from build123d import *

# Parameters (mm, degrees)
F0_W         = 166.2
F0_H         = 100.6
F1_DEPTH     = 5.96
F2_DEPTH     = 0.7
F3_W         = 15
F3_H         = 8
F4_DEPTH     = 2.5
F5_T4_DEPTH  = 33.7168298797
F5_T9_DEPTH  = 33.7168298797
F5_T14_DEPTH = 33.7168298797
F5_T19_DEPTH = 33.7168298797
F5_T24_DEPTH = 33.7168298797
F5_T29_DEPTH = 33.7168298797
F5_T34_DEPTH = 33.7168298797
F5_T39_DEPTH = 33.7168298797
F6_D         = 2.5
F6_DEPTH     = 2.501


# Not quite as in the source:
# - a fillet or chamfer that OpenCascade refuses, or shapes differently, is made with other operations: its cross-section is extruded or revolved along the edge and cut away or added


with BuildPart() as f1:
    # F0 (on Front) → F1 (new body)
    with BuildSketch(Plane.XZ):
        with Locations((-1.49, -1.55)):
            Rectangle(F0_W, F0_H)
    extrude(amount=F1_DEPTH)

    # F0 (on Front) → F2 (join)
    with BuildSketch(Plane.XZ):
        with BuildLine():
            ThreePointArc((-96.48, -47.5), (-94.1720014358, -53.0720014358), (-88.6, -55.38))
            Line((-88.6, -55.38), (88.6, -55.38))
            ThreePointArc((88.6, -55.38), (94.1720014357, -53.0720014357), (96.48, -47.5))
            Line((96.48, -47.5), (96.48, 47.5))
            ThreePointArc((96.48, 47.5), (94.1720014358, 53.0720014358), (88.6, 55.38))
            Line((88.6, 55.38), (-88.6, 55.38))
            ThreePointArc((-88.6, 55.38), (-94.1720014357, 53.0720014357), (-96.48, 47.5))
            Line((-96.48, 47.5), (-96.48, -47.5))
        make_face()
        with Locations((-1.49, -1.55)):
            Rectangle(F0_W, F0_H, mode=Mode.SUBTRACT)
    extrude(amount=F2_DEPTH)

    # F3 (on face) → F4 (join)
    with BuildSketch(Plane.XZ.offset(5.96)):
        with Locations((-64.59, 33.8)):
            Rectangle(F3_W, F3_H)
        with Locations((-64.59, -31.85)):
            Rectangle(F3_W, F3_H)
        with Locations((61.61, -31.85)):
            Rectangle(F3_W, F3_H)
        with Locations((61.61, 33.8)):
            Rectangle(F3_W, F3_H)
    extrude(amount=F4_DEPTH)

    # F5: chamfer of 5 on 8 edges, made by hand


with BuildPart() as f5_tool2:
    # F5_s3 → F5_t4 (new body)
    with BuildSketch(Plane.XY.offset(50.6584149398)):
        Polygon((-72.09, -3.46), (-67.09, -8.46), (-72.09, -8.46), align=None)
    extrude(amount=-F5_T4_DEPTH)

    split(bisect_by=Plane.XZ.offset(5.96), keep=Keep.TOP)


with BuildPart() as f1_1:
    add(f1.part)

    # F5_t1: cut F5_tool2
    add(f5_tool2.part, mode=Mode.SUBTRACT)


with BuildPart() as f5_tool7:
    # F5_s8 → F5_t9 (new body)
    with BuildSketch(Plane.XY.offset(16.9415850602)):
        Polygon((-57.09, -3.46), (-62.09, -8.46), (-57.09, -8.46), align=None)
    extrude(amount=F5_T9_DEPTH)

    split(bisect_by=Plane.XZ.offset(5.96), keep=Keep.TOP)


with BuildPart() as f1_2:
    add(f1_1.part)

    # F5_t6: cut F5_tool7
    add(f5_tool7.part, mode=Mode.SUBTRACT)


with BuildPart() as f5_tool12:
    # F5_s13 → F5_t14 (new body)
    with BuildSketch(Plane.XY.offset(-14.9915850602)):
        Polygon((-72.09, -3.46), (-67.09, -8.46), (-72.09, -8.46), align=None)
    extrude(amount=-F5_T14_DEPTH)

    split(bisect_by=Plane.XZ.offset(5.96), keep=Keep.TOP)


with BuildPart() as f1_3:
    add(f1_2.part)

    # F5_t11: cut F5_tool12
    add(f5_tool12.part, mode=Mode.SUBTRACT)


with BuildPart() as f5_tool17:
    # F5_s18 → F5_t19 (new body)
    with BuildSketch(Plane.XY.offset(-48.7084149398)):
        Polygon((-57.09, -3.46), (-62.09, -8.46), (-57.09, -8.46), align=None)
    extrude(amount=F5_T19_DEPTH)

    split(bisect_by=Plane.XZ.offset(5.96), keep=Keep.TOP)


with BuildPart() as f1_4:
    add(f1_3.part)

    # F5_t16: cut F5_tool17
    add(f5_tool17.part, mode=Mode.SUBTRACT)


with BuildPart() as f5_tool22:
    # F5_s23 → F5_t24 (new body)
    with BuildSketch(Plane.XY.offset(50.6584149398)):
        Polygon((54.11, -3.46), (59.11, -8.46), (54.11, -8.46), align=None)
    extrude(amount=-F5_T24_DEPTH)

    split(bisect_by=Plane.XZ.offset(5.96), keep=Keep.TOP)


with BuildPart() as f1_5:
    add(f1_4.part)

    # F5_t21: cut F5_tool22
    add(f5_tool22.part, mode=Mode.SUBTRACT)


with BuildPart() as f5_tool27:
    # F5_s28 → F5_t29 (new body)
    with BuildSketch(Plane.XY.offset(16.9415850602)):
        Polygon((69.11, -3.46), (64.11, -8.46), (69.11, -8.46), align=None)
    extrude(amount=F5_T29_DEPTH)

    split(bisect_by=Plane.XZ.offset(5.96), keep=Keep.TOP)


with BuildPart() as f1_6:
    add(f1_5.part)

    # F5_t26: cut F5_tool27
    add(f5_tool27.part, mode=Mode.SUBTRACT)


with BuildPart() as f5_tool32:
    # F5_s33 → F5_t34 (new body)
    with BuildSketch(Plane.XY.offset(-14.9915850602)):
        Polygon((54.11, -3.46), (59.11, -8.46), (54.11, -8.46), align=None)
    extrude(amount=-F5_T34_DEPTH)

    split(bisect_by=Plane.XZ.offset(5.96), keep=Keep.TOP)


with BuildPart() as f1_7:
    add(f1_6.part)

    # F5_t31: cut F5_tool32
    add(f5_tool32.part, mode=Mode.SUBTRACT)


with BuildPart() as f5_tool37:
    # F5_s38 → F5_t39 (new body)
    with BuildSketch(Plane.XY.offset(-48.7084149398)):
        Polygon((69.11, -3.46), (64.11, -8.46), (69.11, -8.46), align=None)
    extrude(amount=F5_T39_DEPTH)

    split(bisect_by=Plane.XZ.offset(5.96), keep=Keep.TOP)


with BuildPart() as f1_8:
    add(f1_7.part)

    # F5_t36: cut F5_tool37
    add(f5_tool37.part, mode=Mode.SUBTRACT)

    # F6 (through all, one way)
    with BuildSketch(Plane(origin=(0, -5.96, 0), x_dir=(1, 0, 0), z_dir=(0, 1, 0))):
        with Locations((-64.59, -33.8), (-64.59, 31.85), (61.61, 31.85), (61.61, -33.8)):
            Circle(F6_D / 2)
    extrude(amount=-F6_DEPTH, mode=Mode.SUBTRACT)


solid = f1_8.part
Can you work these out from the model? Positions are in its coordinate system, mm. A direction names the side the tool comes from. Coordinates: 2 decimals unless noted, no trailing zeros. Write each loop counter-clockwise with the first axis right and the second up, starting at its lowest first coordinate (ties: lowest second). Pieces come first, ordered by that corner, then holes.
Q1. Please list where these lines run through material, in increasing order: L1, parallel to Z at x = -64.59, y = -7.7; L2, parallel to Z at x = 26.5, y = -4.5; L3, parallel to Y at x = -33, z = -7.5.
Results found:
L1: z = -35.85 to -33.1, -30.6 to -27.85, 29.8 to 32.55, 35.05 to 37.8
L2: z = -51.85 to 48.75
L3: y = -5.96 to 0
Q2. Imagine slicing it at C-C, the plane y = -2.75. List the corners of the cut face in (x, z) for me, plus the area to 3 significant figures.
Results found:
outline: (-84.59, -51.85) - (81.61, -51.85) - (81.61, 48.75) - (-84.59, 48.75) - close
area: 16,700 mm2
Q3. Imagine slicing it at B-B, the plane z = -11. List the corners of the cut face in (x, y) for me.
Results found:
outline: (-96.48, -0.7) - (-84.59, -0.7) - (-84.59, -5.96) - (81.61, -5.96) - (81.61, -0.7) - (96.48, -0.7) - (96.48, 0) - (-96.48, 0) - close
Q4. For P1, Ø1.5, axis at x = -41, y = -5.5, coming from the -Z side; P2, Ø6, axis at x = -54.5, z = -14, coming from the -Y side; P3, Ø3, axis at y = -5, z = 29.5, coming from the +X side, each with a flat end and sliding along its axis, tell me the tip position at first contact or that it passes through.
Results found:
P1: stops at z = -51.85
P2: stops at y = -5.96
P3: stops at x = 81.61
Q5. Which directions (+Z, -Z, +X, -X, +Y, -Y) give clear straight access to the entire face, cutting with the end or side of a thin tool? Please do faces 1 (the face through (-3, -3, 48.75)), 2 (the face through (81.61, -3, -2)), 3 (the face through (-84.59, -3, -2)), 4 (the face through (-3, -3, -51.85)).
Results found:
face 1: +Z, +X, -X, -Y
face 2: +Z, -Z, +X, -Y
face 3: +Z, -Z, -X, -Y
face 4: -Z, +X, -X, -Y
Q6. Imagine slicing it at A-A, the plane x = 8. List the corners of the cut face in (y, z) for me.
Results found:
outline: (-5.96, -51.85) - (-0.7, -51.85) - (-0.7, -55.38) - (0, -55.38) - (0, 55.38) - (-0.7, 55.38) - (-0.7, 48.75) - (-5.96, 48.75) - close
